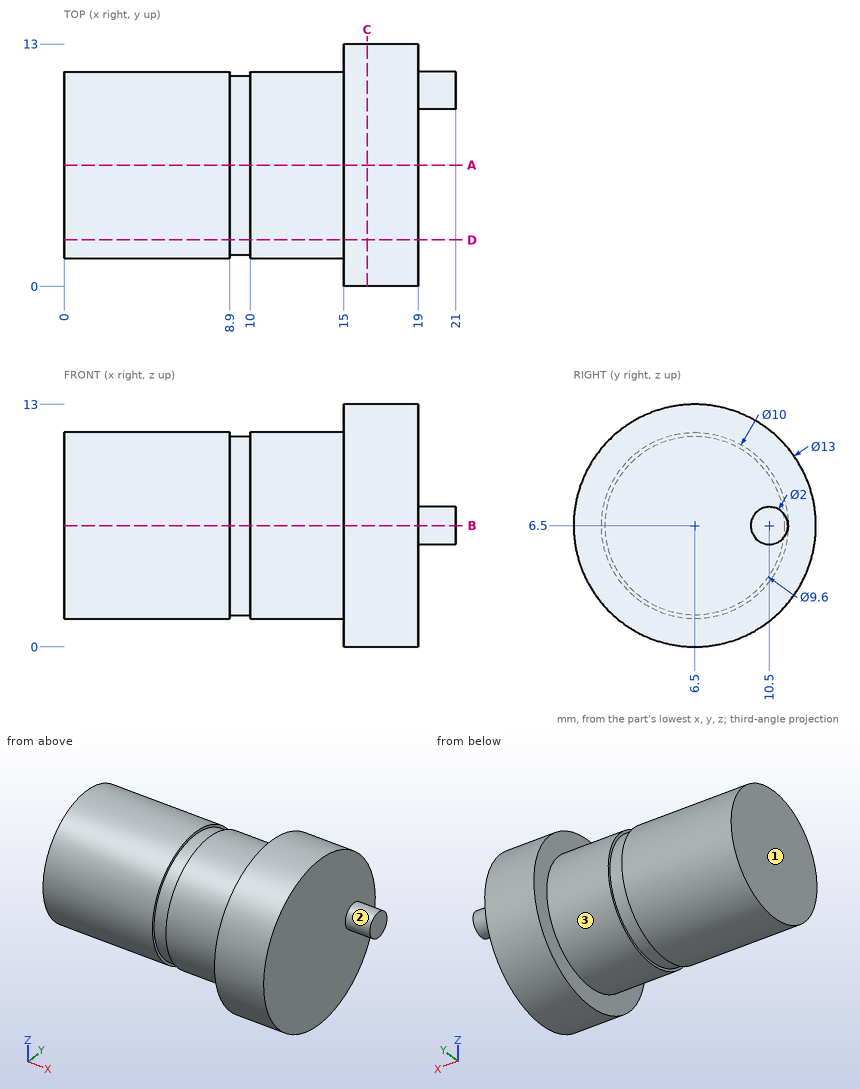
Drawing for the job (mm, zero at the part's lowest x, y, z). A direction names the side the tool comes from. Coordinates: 2 decimals unless noted, no trailing zeros. Order: outer loops, then holes, each group sorted by start corner. A loop starts at its lowest first (then second) coordinate and runs counter-clockwise, first axis right, second up. Notation, with made-up numbers: (-40, 70) -> (11, 70) arc R29 ccw to (11, 94) -> close; hole circle Ø3 at (71, 12.5). An arc over 180 degrees is marked (long way). Answer in a Markdown table with one row per item.
1) Band-saw the part on A-A (y = 6.5). List the corners of the cut face in (x, z), and give its area (3 significant figures).
Check values:
| item | result |
|---|---|
| outline | (0, 1.5) -> (8.9, 1.5) -> (8.9, 1.7) -> (10, 1.7) -> (10, 1.5) -> (15, 1.5) -> (15, 0) -> (19, 0) -> (19, 13) -> (15, 13) -> (15, 11.5) -> (10, 11.5) -> (10, 11.3) -> (8.9, 11.3) -> (8.9, 11.5) -> (0, 11.5) -> close |
| area | 202 mm2 |
2) Which spindle directions (+Z, -Z, +X, -X, +Y, -Y) get a long thin tool onto all of the face, cutting with end or side? Do the marked faces 1, 2 and 3. Say none if no direction does.
Check values:
| item | result |
|---|---|
| face 1 | +Z, -Z, -X, +Y, -Y |
| face 2 | +X |
| face 3 | -X |
3) Band-saw the part on B-B (z = 6.5). List the corners of the cut face in (x, y), and give its area (3 significant figures).
Check values:
| item | result |
|---|---|
| outline | (0, 1.5) -> (8.9, 1.5) -> (8.9, 1.7) -> (10, 1.7) -> (10, 1.5) -> (15, 1.5) -> (15, 0) -> (19, 0) -> (19, 9.5) -> (21, 9.5) -> (21, 11.5) -> (19, 11.5) -> (19, 13) -> (15, 13) -> (15, 11.5) -> (10, 11.5) -> (10, 11.3) -> (8.9, 11.3) -> (8.9, 11.5) -> (0, 11.5) -> close |
| area | 206 mm2 |
4) Band-saw the part on D-D (y = 2.5). List the corners of the cut face in (x, z).
Check values:
| item | result |
|---|---|
| outline | (0, 3.5) -> (8.9, 3.5) -> (8.9, 3.85) -> (10, 3.85) -> (10, 3.5) -> (15, 3.5) -> (15, 1.38) -> (19, 1.38) -> (19, 11.62) -> (15, 11.62) -> (15, 9.5) -> (10, 9.5) -> (10, 9.15) -> (8.9, 9.15) -> (8.9, 9.5) -> (0, 9.5) -> close |
5) Band-saw the part on C-C (x = 16.25). List the corners of the cut face in (y, z), and give its area (3 significant figures).
Check values:
| item | result |
|---|---|
| outline | circle Ø13 at (6.5, 6.5) |
| area | 133 mm2 |
6) Flat gauge pins, fed straight in: P1, Ø3, axis at y = 2, z = 5, coming from the +X side; P2, Ø1.5, axis at x = 4.5, y = 6.5, coming from the -Z side; P3, Ø2, axis at x = 18.5, y = 5, coming from the -Z side. Where does each tip first touch, or does it go through?
Check values:
| item | result |
|---|---|
| P1 | x = 19 |
| P2 | z = 1.5 |
| P3 | z = 0.02 |
7) Drill centre lines: line 1 (Y direction, x = 11.25, z = 6.5); line 2 (X direction, y = 2, z = 8); line 3 (Y direction, x = 17.25, z = 0.75). Where is each one in solid material? Low to high.
Check values:
| item | result |
|---|---|
| line 1 | 1.5 to 11.5 |
| line 2 | 0 to 19 |
| line 3 | 3.47 to 9.53 |
